from build123d import *

# Parameters (mm, degrees)
F0_W     = 30
F0_H     = 50
F1_DEPTH = 3
F2_W     = 15
F2_H     = 3
F3_DEPTH = 17
F4_W     = 15
F4_H     = 3
F5_DEPTH = 55
F6_W     = 15
F6_H     = 35
F7_DEPTH = 3


with BuildPart() as f1:
    # F0 (on Front) → F1 (new body)
    with BuildSketch(Plane.XZ):
        Rectangle(F0_W, F0_H)
        with BuildLine():
            ThreePointArc((-12.25, 15), (-10, 17.25), (-7.75, 15))
            Line((-7.75, 15), (-7.75, 5))
            ThreePointArc((-7.75, 5), (-10, 2.75), (-12.25, 5))
            Line((-12.25, 5), (-12.25, 15))
        make_face(mode=Mode.SUBTRACT)
        with BuildLine():
            Line((12.25, 15), (12.25, 5))
            ThreePointArc((12.25, 5), (10, 2.75), (7.75, 5))
            Line((7.75, 5), (7.75, 15))
            ThreePointArc((7.75, 15), (10, 17.25), (12.25, 15))
        make_face(mode=Mode.SUBTRACT)
    extrude(amount=F1_DEPTH)

    # F2 (on face) → F3 (join)
    with BuildSketch(Plane.XZ.offset(3)):
        with Locations((0, -23.5)):
            Rectangle(F2_W, F2_H)
    extrude(amount=F3_DEPTH)

    # F4 (on face) → F5 (join)
    with BuildSketch(Plane(origin=(0, 0, -25), x_dir=(1, 0, 0), z_dir=(0, 0, -1))):
        with Locations((0, 18.5)):
            Rectangle(F4_W, F4_H)
    extrude(amount=F5_DEPTH)

    # F6 (on face) → F7 (join)
    with BuildSketch(Plane(origin=(0, 0, -80), x_dir=(1, 0, 0), z_dir=(0, 0, -1))):
        with Locations((0, 2.5)):
            Rectangle(F6_W, F6_H)
        with BuildLine():
            ThreePointArc((-3.25, 10), (0, 13.25), (3.25, 10))
            Line((3.25, 10), (3.25, -8))
            ThreePointArc((3.25, -8), (0, -11.25), (-3.25, -8))
            Line((-3.25, -8), (-3.25, 10))
        make_face(mode=Mode.SUBTRACT)
    extrude(amount=-F7_DEPTH)


solid = f1.part
Work out the finished part from the listing and answer in its coordinate system (mm). A direction names the side the tool comes from. Coordinates: 2 decimals unless noted, no trailing zeros. Order: outer loops, then holes, each group sorted by start corner. A loop starts at its lowest first (then second) coordinate and runs counter-clockwise, first axis right, second up. Notation, with made-up numbers: (36, -5.5) - (57, -5.5) arc R16 cw to (57, 10.5) - close; hole circle Ø10 at (23.5, 33.5). An arc over 180 degrees is marked (long way). Put each result on its own line as item: value. Start each with the question number.
1) Find section D-D (z = 0). Give the vertices of the cut face in (x, y).
2) Flat-ended cylindrical pins translate along their axes: pin 1 (9 mm diameter, centred on x = 2, z = -3, fed in from +Y); pin 2 (8 mm diameter, centred on x = -5, y = 7, fed in from +Z); pin 3 (12 mm diameter, centred on y = -15.5, z = -32, fed in from -X). Find the tip coordinate at first contact, or state that the pin passes through.
3) Find section B-B (y = 1). Give the vertices of the cut face in (x, z).
4) Find the intervals of material crossed by line 1 (Z direction, x = 7, y = -4); line 2 (Y direction, x = 9.25, z = -23); line 3 (Y direction, x = -6.5, z = -30.5), in increasing order. Write a range as from..to.
5) Find section C-C (x = 0). Give the vertices of the cut face in (y, z), plus the area to 4 significant figures.
6) For a pull along X with two mould halves and no side action, classify faces 1 (the cylindrical face through (-9.95, -1.48, 2.75)), 2 (the flat face through (-7.5, -18, -55)), 3 (the flat face through (12.25, -1, 10)), 4 (the flat face through (0, -17, -51)) as released by +X, released by -X, zero draft, split by the parting line, or undercut.
7) For faces 5 (the flat face through (0, -11, -22)), 6 (the flat face through (-3.25, -1, -79)), 7 (the flat face through (-3.44, -1.22, -77)), 8 (the cylindrical face through (0.07, 11.25, -78.52)), determine the directions among +Z, -Z, +X, -X, +Y, -Y from which every point of the face is accessible in a straight line to the end or side of a thin tool.
8) Find section A-A (x = -10). Give the vertices of the cut face in (y, z).
Results list:
1. outline: (-15, -3) - (15, -3) - (15, 0) - (-15, 0) - close
2. pin 1: stops at y = 0
2. pin 2: stops at z = -77
2. pin 3: stops at x = -7.5
3. outline: (-7.5, -80) - (-3.25, -80) - (-3.25, -77) - (-7.5, -77) - close; (3.25, -80) - (7.5, -80) - (7.5, -77) - (3.25, -77) - close
4. line 1: z = -80..-77, -25..-22
4. line 2: y = -3..0
4. line 3: y = -20..-17
5. outline: (-20, -80) - (-13.25, -80) - (-13.25, -77) - (-17, -77) - (-17, -25) - (0, -25) - (0, 25) - (-3, 25) - (-3, -22) - (-20, -22) - close; (11.25, -80) - (15, -80) - (15, -77) - (11.25, -77) - close
5. area: 388.5 mm^2
6. face 1: undercut
6. face 2: released by -X
6. face 3: undercut
6. face 4: zero draft
7. face 5: +Z, +X, -X, -Y
7. face 6: -Z
7. face 7: +X, -X, +Y
7. face 8: +Z, -Z
8. outline: (-3, -25) - (0, -25) - (0, 2.75) - (-3, 2.75) - close; (-3, 17.25) - (0, 17.25) - (0, 25) - (-3, 25) - close
